```python
from build123d import *

# Parameters (mm, degrees)
SKETCH2_W                = 10.16
SKETCH2_H                = 4.572
BASE_EXTRUDE_DEPTH       = 14.732
CUT_EXTRUDE1_DEPTH       = 1
CUT_EXTRUDE1_DEPTH_BACK  = 11.16
CUT_EXTRUDE4_DEPTH       = 0.0254
CUT_EXTRUDE5_DEPTH       = 0.0254
CUT_EXTRUDE6_DEPTH       = 0.0254
BOSS_EXTRUDE_THIN1_DEPTH = 0.4064
LPATTERN2_COUNT          = 4
LPATTERN2_PITCH          = 2.54
BOSS_EXTRUDE_THIN2_DEPTH = 0.4064
LPATTERN3_COUNT          = 3
LPATTERN3_PITCH          = 2.54
SKETCH4_R                = 1.905
CUT_EXTRUDE2_DEPTH       = 14.732


with BuildPart() as part:
    # Sketch2 → Base-Extrude (new body)
    with BuildSketch(Plane(origin=(0, 6.35, 0), x_dir=(-1, 0, 0), z_dir=(0, 1, 0))):
        with Locations((-3.81, -5.3086)):
            Rectangle(SKETCH2_W, SKETCH2_H)
    extrude(amount=BASE_EXTRUDE_DEPTH)

    # Sketch3 → Cut-Extrude1 (cut, two sides)
    with BuildSketch(Plane.ZY.offset(1.27)) as cut_extrude1_sk:
        Polygon((-6.3246, 21.082), (-6.3246, 14.986), (-3.0226, 14.478), (-3.0226, 21.082), align=None)
    extrude(amount=CUT_EXTRUDE1_DEPTH, mode=Mode.SUBTRACT)
    extrude(cut_extrude1_sk.sketch, amount=-CUT_EXTRUDE1_DEPTH_BACK, mode=Mode.SUBTRACT)

    # Sketch5 → Cut-Extrude4 (cut)
    with BuildSketch(Plane.ZY.offset(1.27)):
        Polygon((-7.5946, 15.181384615), (-3.0226, 14.478), (-3.0226, 6.35), (-7.5946, 6.35), align=None)
    extrude(amount=-CUT_EXTRUDE4_DEPTH, mode=Mode.SUBTRACT)

    # Sketch6 → Cut-Extrude5 (cut)
    with BuildSketch(Plane(origin=(8.89, 0, 0), x_dir=(0, 0, -1), z_dir=(1, 0, 0))):
        Polygon((3.0226, 14.478), (7.5946, 15.181384615), (7.5946, 6.35), (3.0226, 6.35), align=None)
    extrude(amount=-CUT_EXTRUDE5_DEPTH, mode=Mode.SUBTRACT)

    # Sketch7 → Cut-Extrude6 (cut)
    with BuildSketch(Plane(origin=(0, 0, -7.5946), x_dir=(-1, 0, 0), z_dir=(0, 0, -1))):
        Polygon((-8.89, 21.082), (-8.89, 15.181384615), (-7.62, 15.181384615), (-7.62, 9.652), (0, 9.652), (0, 15.181384615), (1.27, 15.181384615), (1.27, 21.082), align=None)
    extrude(amount=-CUT_EXTRUDE6_DEPTH, mode=Mode.SUBTRACT)

    # Sketch9 → Boss-Extrude-Thin1 (add, symmetric)
    with BuildSketch(Plane(origin=(0, 0, 0), x_dir=(0, 0, -1), z_dir=(1, 0, 0))):
        with BuildLine():
            Line((5.1562, 6.35), (5.1562, 3.7846))
            ThreePointArc((5.1562, 3.7846), (5.07392687, 3.499994822), (4.852487561, 3.303186265))
            Line((4.852487561, 3.303186265), (0.335437388, 1.14805408))
            ThreePointArc((0.335437388, 1.14805408), (-0.075807043, 0.782552474), (-0.2286, 0.254))
            Line((-0.2286, 0.254), (-0.2286, -2.54))
            Line((-0.2286, -2.54), (0.2286, -2.54))
            Line((0.2286, -2.54), (0.2286, 0.254))
            ThreePointArc((0.2286, 0.254), (0.31087313, 0.538605178), (0.532312439, 0.735413735))
            Line((0.532312439, 0.735413735), (5.049362612, 2.89054592))
            ThreePointArc((5.049362612, 2.89054592), (5.460607043, 3.256047526), (5.6134, 3.7846))
            Line((5.6134, 3.7846), (5.6134, 6.35))
            Line((5.6134, 6.35), (5.1562, 6.35))
        make_face()
    boss_extrude_thin1 = extrude(amount=BOSS_EXTRUDE_THIN1_DEPTH, both=True)

    # LPattern2: Boss-Extrude-Thin1 ×4
    with Locations(*[(i * LPATTERN2_PITCH, 0, 0) for i in range(1, LPATTERN2_COUNT)]):
        add(boss_extrude_thin1)

    # Sketch10 → Boss-Extrude-Thin2 (add, symmetric)
    with BuildSketch(Plane(origin=(1.27, 0, 0), x_dir=(0, 0, -1), z_dir=(1, 0, 0))):
        with BuildLine():
            Line((5.08, 6.35), (5.08, 3.433803724))
            ThreePointArc((5.08, 3.433803724), (5.065314035, 3.309500424), (5.022064828, 3.192041946))
            Line((5.022064828, 3.192041946), (3.66359389, 0.520382434))
            ThreePointArc((3.66359389, 0.520382434), (3.583273936, 0.302245261), (3.556, 0.071396276))
            Line((3.556, 0.071396276), (3.556, -5.588))
            Line((3.556, -5.588), (4.0132, -5.588))
            Line((4.0132, -5.588), (4.0132, 0.071396276))
            ThreePointArc((4.0132, 0.071396276), (4.027885965, 0.195699576), (4.071135172, 0.313158054))
            Line((4.071135172, 0.313158054), (5.42960611, 2.984817566))
            ThreePointArc((5.42960611, 2.984817566), (5.509926064, 3.202954739), (5.5372, 3.433803724))
            Line((5.5372, 3.433803724), (5.5372, 6.35))
            Line((5.5372, 6.35), (5.08, 6.35))
        make_face()
    boss_extrude_thin2 = extrude(amount=BOSS_EXTRUDE_THIN2_DEPTH, both=True)

    # LPattern3: Boss-Extrude-Thin2 ×3
    with Locations(*[(i * LPATTERN3_PITCH, 0, 0) for i in range(1, LPATTERN3_COUNT)]):
        add(boss_extrude_thin2)

    # Sketch4 → Cut-Extrude2 (cut)
    with BuildSketch(Plane.XY.offset(-6.3246)):
        with Locations((3.81, 18.415)):
            Circle(SKETCH4_R)
    extrude(amount=-CUT_EXTRUDE2_DEPTH, mode=Mode.SUBTRACT)


solid = part.part
```
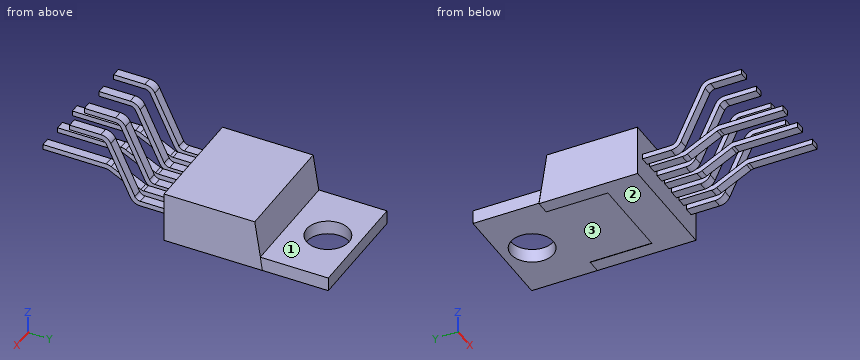
Part model, mm, in its own coordinate system. Face numbers are marked on the shaded views. A direction names the side the tool comes from. Round coordinates to 2 decimals unless told otherwise and drop trailing zeros. Loops run counter-clockwise (first coordinate to the right, second up) from the corner with the lowest first, then second, coordinate; pieces in that order, holes last.
Item 1: 3-axis set-ups, long thin cutter, end or side, ignore diameter. For the marked faces 1, 2 and 3: which of +Z, -Z, +X, -X, +Y, -Y reach the whole face in a straight line?
Item 2: Drill centre lines: line 1 (X direction, y = 1, z = -0.5); line 2 (Y direction, x = 3.81, z = -7.25); line 3 (Z direction, x = 5.75, y = 19.75). Where is each one in solid material? Low to high.
Item 3: Cut at A-A, the plane y = -1. Give the cut face in (x, z).
Item 4: Drop flat-ended pins along their axis: P1, Ø3, axis at y = 2, z = -6, coming from the +X side; P2, Ø3, axis at x = 3.5, y = 18, coming from the +Z side; P3, Ø0.9, axis at x = 2.5, y = 5, coming from the +Z side. Give the stop position or say it passes through.
Item 5: Cut at B-B, the plane z = -2.5. Give the cut face in (x, y).
A:
1. face 1: +Z, +X, -X, +Y
1. face 2: -Z, +X, -X, +Y, -Y
1. face 3: -Z, +Y
2. line 1: x = -0.41 to 0.41, 2.13 to 2.95, 4.67 to 5.49, 7.21 to 8.03
2. line 2: y = 6.35 to 16.51, 20.32 to 21.08
2. line 3: z = -7.57 to -6.32
3. outline: (-0.41, -0.23) - (0.41, -0.23) - (0.41, 0.23) - (-0.41, 0.23) - close; (0.86, -4.01) - (1.68, -4.01) - (1.68, -3.56) - (0.86, -3.56) - close; (2.13, -0.23) - (2.95, -0.23) - (2.95, 0.23) - (2.13, 0.23) - close; (3.4, -4.01) - (4.22, -4.01) - (4.22, -3.56) - (3.4, -3.56) - close; (4.67, -0.23) - (5.49, -0.23) - (5.49, 0.23) - (4.67, 0.23) - close; (5.94, -4.01) - (6.76, -4.01) - (6.76, -3.56) - (5.94, -3.56) - close; (7.21, -0.23) - (8.03, -0.23) - (8.03, 0.23) - (7.21, 0.23) - close
4. P1: stops at x = 8.03
4. P2: stops at z = -6.32
4. P3: stops at z = -5.16
5. outline: (-0.41, 1.67) - (0.41, 1.67) - (0.41, 2.18) - (-0.41, 2.18) - close; (2.13, 1.67) - (2.95, 1.67) - (2.95, 2.18) - (2.13, 2.18) - close; (4.67, 1.67) - (5.49, 1.67) - (5.49, 2.18) - (4.67, 2.18) - close; (7.21, 1.67) - (8.03, 1.67) - (8.03, 2.18) - (7.21, 2.18) - close
